Verification items for the finished model (mm, model axes). Round coordinates to 2 decimals unless told otherwise and drop trailing zeros. Loops run counter-clockwise (first coordinate to the right, second up) from the corner with the lowest first, then second, coordinate; pieces in that order, holes last. Notation, with made-up numbers: M -20,-34 L 28,-34 A22 cw 28,-3 Z; hole C 69,-13.75 d8. An arc over 180 degrees is marked long. One line per item, written item: value.
from build123d import *

# Parameters (mm, degrees)
F0_W     = 70
F0_H     = 20
F1_DEPTH = 10
F3_D     = 6.8
F3_DEPTH = 15.75
F3_TIP   = 2.0429261047


with BuildPart() as f1:
    # F0 (on Top) → F1 (new body)
    with BuildSketch(Plane.XY):
        with Locations((9.6113178879, -1.2831067624)):
            Rectangle(F0_W, F0_H)
    extrude(amount=F1_DEPTH)

    # F3
    with Locations(Plane.XY.offset(10)):
        with Locations((27.1113178879, -1.2831067624), (9.6113178879, -1.2831067624), (-7.8886821121, -1.2831067624)):
            Hole(F3_D / 2, depth=F3_DEPTH)
            with Locations((0, 0, -(F3_DEPTH + F3_TIP / 2))):  # 118° drill point
                Cone(0, F3_D / 2, F3_TIP, mode=Mode.SUBTRACT)


solid = f1.part
(1) Sectioned sample at B-B on x = -9. Enter the section's corners in (y, z).
Completed:
outline: M -11.28,0 L -4.5,0 L -4.5,10 L -11.28,10 Z; M 1.93,0 L 8.72,0 L 8.72,10 L 1.93,10 Z
(2) Sectioned sample at A-A on y = -3. Enter the section's corners in (x, z), and give its area (3 significant figures).
Completed:
outline: M -25.39,0 L -10.82,0 L -10.82,10 L -25.39,10 Z; M -4.95,0 L 6.68,0 L 6.68,10 L -4.95,10 Z; M 12.55,0 L 24.18,0 L 24.18,10 L 12.55,10 Z; M 30.05,0 L 44.61,0 L 44.61,10 L 30.05,10 Z
area: 524 mm^2
(3) Mould release check, pull along X, two halves, no side actions. Record for faces 1 (the face through (-25.389, -1, 5)), 2 (the face through (9, 3, 10)), 3 (the face through (23.87, -0.26, 4.93)): +X half, -X half, draft (parallel to the pull), parting line (faces both ways), or undercut.
Completed:
face 1: -X half
face 2: draft
face 3: undercut
(4) Depth check by flat-ended pin: pin 1 Ø2 at (x, y) = (34.5, 3.5) entering from -Z. Enter the tip coordinate at first touch or a pass-through.
Completed:
pin 1: stops at z = 0
(5) Sectioned sample at C-C on z = 6.75. Enter the section's corners in (x, y).
Completed:
outline: M -25.39,-11.28 L 44.61,-11.28 L 44.61,8.72 L -25.39,8.72 Z; hole C -7.89,-1.28 d6.8; hole C 9.61,-1.28 d6.8; hole C 27.11,-1.28 d6.8
(6) Thickness scan on L1, parallel to X at y = -2.75, z = 8; L2, parallel to X at y = -4, z = 7.25; L3, parallel to Y at x = -5, z = 2. Record the ranges inside material, lowest first. Write a range as from..to.
Completed:
L1: x = -25.39..-10.96, -4.82..6.54, 12.68..24.04, 30.18..44.61
L2: x = -25.39..-9.93, -5.84..7.57, 11.66..25.07, 29.16..44.61
L3: y = -11.28..-3.08, 0.51..8.72
(7) Sectioned sample at D-D on x = 25. Enter the section's corners in (y, z).
Completed:
outline: M -11.28,0 L -3.95,0 L -3.95,10 L -11.28,10 Z; M 1.38,0 L 8.72,0 L 8.72,10 L 1.38,10 Z
